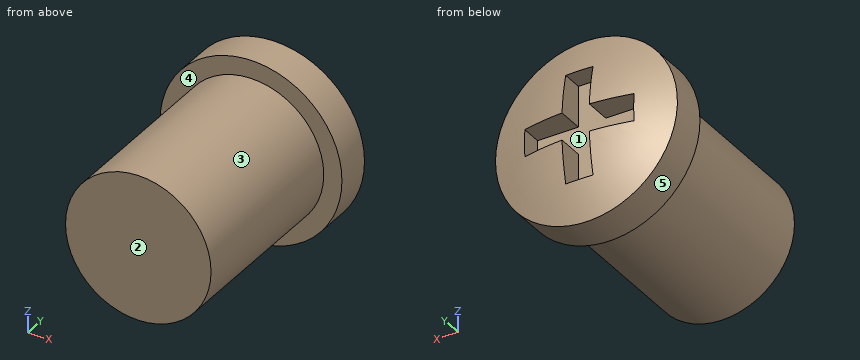
```python
from build123d import *

# Parameters (mm, degrees)
SKETCH1_R           = 2
BOSS_EXTRUDE1_DEPTH = 5
SKETCH2_R           = 2.5
BOSS_EXTRUDE2_DEPTH = 1
DOME1_FACE_RADIUS   = 2.5
DOME1_HEIGHT        = 0.5
SKETCH3_W           = 1.125
SKETCH3_H           = 0.75
SKETCH3_W_2         = 0.75
SKETCH3_H_2         = 1.125
CUT_EXTRUDE1_DEPTH  = 0.75


with BuildPart() as part:
    # Sketch1 → Boss-Extrude1 (new body)
    with BuildSketch(Plane(origin=(0, 0, 0), x_dir=(1, 0, 0), z_dir=(0, 1, 0))):
        Circle(SKETCH1_R)
    extrude(amount=BOSS_EXTRUDE1_DEPTH)

    # Sketch2 → Boss-Extrude2 (add)
    with BuildSketch(Plane(origin=(0, 5, 0), x_dir=(1, 0, 0), z_dir=(0, 1, 0))):
        Circle(SKETCH2_R)
    extrude(amount=BOSS_EXTRUDE2_DEPTH)

    # Dome1: a dome of height H over a round flat face of radius A is a cap of a sphere of radius (A * A + H * H) / (2 * H)
    dome1_r = (DOME1_FACE_RADIUS * DOME1_FACE_RADIUS + DOME1_HEIGHT * DOME1_HEIGHT) / (2 * DOME1_HEIGHT)
    dome1_base = Plane((0, 6, 0), z_dir=(0, 1, 0))
    with Locations(dome1_base.offset(DOME1_HEIGHT - dome1_r)):
        dome1_ball = Sphere(dome1_r, mode=Mode.PRIVATE)
    add(split(dome1_ball, bisect_by=dome1_base, keep=Keep.TOP, mode=Mode.PRIVATE))

    # Sketch3 → Cut-Extrude1 (cut)
    with BuildSketch(Plane(origin=(0, 6.5, 0), x_dir=(1, 0, 0), z_dir=(0, 1, 0))):
        with Locations((-0.9375, 0)):
            Rectangle(SKETCH3_W, SKETCH3_H)
        Rectangle(SKETCH3_W_2, SKETCH3_H)
        with Locations((0, 0.9375)):
            Rectangle(SKETCH3_W_2, SKETCH3_H_2)
        with Locations((0.9375, 0)):
            Rectangle(SKETCH3_W, SKETCH3_H)
        with Locations((0, -0.9375)):
            Rectangle(SKETCH3_W_2, SKETCH3_H_2)
    extrude(amount=-CUT_EXTRUDE1_DEPTH, mode=Mode.SUBTRACT)


solid = part.part
```
Can you work these out from the model? Positions are in its coordinate system, mm. Face numbers are marked on the shaded views. A direction names the side the tool comes from. Coordinates: 2 decimals unless noted, no trailing zeros. Loops run counter-clockwise (first coordinate to the right, second up) from the corner with the lowest first, then second, coordinate; pieces in that order, holes last. Notation, with made-up numbers: (-1.75, 41) -> (5.25, 41) arc R14 cw to (5.25, 47) -> close; hole circle Ø6 at (80.5, 79). An arc over 180 degrees is marked (long way). Answer as a JSON object with one key per item and string values.
1) For the marked faces 4 and 5, which set-ups out of +Z, -Z, +X, -X, +Y, -Y let a thin tool reach every point of the face, with its end or its side?
Results:
{"face 4": "-Y", "face 5": "+Y, -Y"}
2) For P1, Ø0.6, axis at y = 6, z = 1, coming from the +X side; P2, Ø0.6, axis at x = 1, y = 6, coming from the -Z side; P3, Ø1.5, axis at x = -0.5, z = -2, coming from the +Y side, each with a flat end and sliding along its axis, tell me the tip position at first contact or that it passes through.
Results:
{"P1": "stops at x = 2.4", "P2": "stops at z = -2.4", "P3": "stops at y = 6.37"}
3) Imagine slicing it at D-D (x = -1.65). Please give me the cut outline in (y, z), then the cut area to 3 significant figures.
Results:
{"outline": "(0, -1.13) -> (5, -1.13) -> (5, -1.88) -> (6, -1.88) arc R6.29 ccw to (6, 1.88) -> (5, 1.88) -> (5, 1.13) -> (0, 1.13) -> close", "area": "15.8 mm^2"}
4) Thinking about a two-plate mould opening in Z: for the marked faces 1, 2 and 3, which applies, pulls with the +Z half, pulls with the -Z half, needs draft (parallel to the pull), parting line crosses it, or undercut?
Results:
{"face 1": "undercut", "face 2": "needs draft", "face 3": "parting line crosses it"}
5) Imagine slicing it at B-B (x = 0). Please give me the cut outline in (y, z).
Results:
{"outline": "(0, -2) -> (5, -2) -> (5, -2.5) -> (6, -2.5) arc R6.5 ccw to (6.32, -1.5) -> (5.75, -1.5) -> (5.75, 1.5) -> (6.32, 1.5) arc R6.5 ccw to (6, 2.5) -> (5, 2.5) -> (5, 2) -> (0, 2) -> close"}
6) If I drill on line 1 (Z direction, x = 0, y = 3); line 2 (X direction, y = 4.5, z = -1.5), over which ranges is the centre line in solid material (lowest first)?
Results:
{"line 1": "z = -2 to 2", "line 2": "x = -1.32 to 1.32"}
7) Imagine slicing it at C-C (y = 0.5). Please give me the cut outline in (x, z), then the cut area to 3 significant figures.
Results:
{"outline": "circle Ø4 at (0, 0)", "area": "12.6 mm^2"}
8) Imagine slicing it at A-A (z = 0). Please give me the cut outline in (x, y).
Results:
{"outline": "(-2.5, 5) -> (-2, 5) -> (-2, 0) -> (2, 0) -> (2, 5) -> (2.5, 5) -> (2.5, 6) arc R6.5 ccw to (1.5, 6.32) -> (1.5, 5.75) -> (-1.5, 5.75) -> (-1.5, 6.32) arc R6.5 ccw to (-2.5, 6) -> close"}
